from build123d import *

# Parameters (mm, degrees)
SKETCH1_R           = 20
BOSS_EXTRUDE1_DEPTH = 3
SKETCH2_W           = 50
SKETCH2_H           = 3
BOSS_EXTRUDE2_DEPTH = 45
SKETCH3_R           = 2
CUT_EXTRUDE1_DEPTH  = 73.835430939


with BuildPart() as part:
    # Sketch1 → Boss-Extrude1 (new body)
    with BuildSketch(Plane.XY):
        with BuildLine():
            Line((-25, 0), (25, 0))
            Line((25, 0), (25, 29))
            ThreePointArc((25, 29), (0, 54), (-25, 29))
            Line((-25, 29), (-25, 0))
        make_face()
        with Locations((0, 29)):
            Circle(SKETCH1_R, mode=Mode.SUBTRACT)
    extrude(amount=BOSS_EXTRUDE1_DEPTH)

    # Sketch2 → Boss-Extrude2 (add)
    with BuildSketch(Plane.XY.offset(3)):
        with Locations((0, -1.5)):
            Rectangle(SKETCH2_W, SKETCH2_H)
    extrude(amount=-BOSS_EXTRUDE2_DEPTH)

    # Sketch3 → Cut-Extrude1 (cut, through all)
    with BuildSketch(Plane(origin=(0, 0, 0), x_dir=(1, 0, 0), z_dir=(0, 1, 0))):
        with Locations(Location((-20, 37, 0), (0, 0, 180))):
            Circle(SKETCH3_R)
        with Locations(Location((-20, 10, 0), (0, 0, 180))):
            Circle(SKETCH3_R)
        with Locations((20, 10)):
            Circle(SKETCH3_R)
        with Locations((20, 37)):
            Circle(SKETCH3_R)
    extrude(amount=-CUT_EXTRUDE1_DEPTH, mode=Mode.SUBTRACT)


solid = part.part
Model file for the job. Use its own axes, mm. A direction names the side the tool comes from. Give positions to 0.01 mm unless a question says otherwise; leave off trailing zeros. Order: outer loops, then holes, each group sorted by start corner. A loop starts at its lowest first (then second) coordinate and runs counter-clockwise, first axis right, second up. Notation, with made-up numbers: M 8,72 L 20,72 A30 cw 20,95 Z; hole C -37.5,20.5 d2. An arc over 180 degrees is marked long. Write item = value, one per line.
Q1. Cut at C-C, the plane y = 32.5. List the corners of the cut face in (x, z), then the cut area to 3 significant figures.
Derived:
outline = M -24.75,0 L -19.69,0 L -19.69,3 L -24.75,3 Z; M 19.69,0 L 24.75,0 L 24.75,3 L 19.69,3 Z
area = 30.4 mm2
Q2. Cut at A-A, the plane z = -37. List the corners of the cut face in (x, y), then the cut area to 3 significant figures.
Derived:
outline = M -25,-3 L -22,-3 L -22,0 L -25,0 Z; M -18,-3 L 18,-3 L 18,0 L -18,0 Z; M 22,-3 L 25,-3 L 25,0 L 22,0 Z
area = 126 mm2
Q3. Tool access for faces 1 (the cylindrical face through (0.55, 53.994, 1.479)), 2 (the flat face through (0, 0, -21)): list every direction of +Z, -Z, +X, -X, +Y, -Y with a clear straight run to the whole face (end or side of a thin tool).
Derived:
face_1 = +Z, -Z, +Y
face_2 = -Z, +X, -X, +Y
Q4. Drill centre lines: line 1 (Z direction, x = -20, y = -1); line 2 (Y direction, x = 0, z = 0.6); line 3 (Z direction, x = -21, y = 21.5). Where is each one in solid material? Low to high. Write a range as [from, to].
Derived:
line_1 = [-42, -39], [-35, -12], [-8, 3]
line_2 = [-3, 9], [49, 54]
line_3 = [0, 3]
Q5. Cut at B-B, the plane x = 0. List the corners of the cut face in (y, z), then the cut area to 3 significant figures.
Derived:
outline = M -3,-42 L 0,-42 L 0,0 L 9,0 L 9,3 L -3,3 Z; M 49,0 L 54,0 L 54,3 L 49,3 Z
area = 177 mm2
Q6. Two-plate mould, pull along X, no slides. Class faces 3 (the cylindrical face through (-18.526, -1.479, -8.648)), 4 (the flat face through (25, -1, -13)), 5 (the flat face through (0, 7, 3)), 6 (the cylindrical face through (-2.6, 48.83, 1.48)): pulls with the +X half, pulls with the -X half, needs draft (parallel to the pull), parting line crosses it, or undercut.
Derived:
face_3 = undercut
face_4 = pulls with the +X half
face_5 = needs draft
face_6 = undercut
Q7. Flat gauge pins, fed straight in: pin 1 (1 mm diameter, centred on x = -10, z = -8, fed in from +Y); pin 2 (12 mm diameter, centred on x = 16, y = 28, fed in from -Z); pin 3 (5 mm diameter, centred on x = -20, z = -10, fed in from -Y). Where does each tip first touch, or does it go through?
Derived:
pin_1 = 0
pin_2 = 0
pin_3 = -3
Q8. Cut at D-D, the plane z = -5. List the corners of the cut face in (x, y).
Derived:
outline = M -25,-3 L 25,-3 L 25,0 L -25,0 Z
